from build123d import *

# Parameters (mm, degrees)
SKETCH3_W                = 25.4
SKETCH3_H                = 25.4
SKETCH3_W_2              = 22.225
SKETCH3_H_2              = 22.225
BOSS_EXTRUDE1_DEPTH      = 76.2
BOSS_EXTRUDE1_DEPTH_BACK = 76.2
SKETCH4_W                = 25.4
SKETCH4_H                = 25.4
SKETCH4_W_2              = 22.225
SKETCH4_H_2              = 22.225
CUT_EXTRUDE1_DEPTH       = 7.9375


with BuildPart() as part:
    # Sketch3 → Boss-Extrude1 (new body, two sides)
    with BuildSketch(Plane.XY) as boss_extrude1_sk:
        Rectangle(SKETCH3_W, SKETCH3_H)
        Rectangle(SKETCH3_W_2, SKETCH3_H_2, mode=Mode.SUBTRACT)
    extrude(amount=BOSS_EXTRUDE1_DEPTH)
    extrude(boss_extrude1_sk.sketch, amount=-BOSS_EXTRUDE1_DEPTH_BACK)

    # Sketch4 → Cut-Extrude1 (cut)
    with BuildSketch(Plane(origin=(0, 0, -76.2), x_dir=(-1, 0, 0), z_dir=(0, 0, -1))):
        Rectangle(SKETCH4_W, SKETCH4_H)
        Rectangle(SKETCH4_W_2, SKETCH4_H_2, mode=Mode.SUBTRACT)
    extrude(amount=-CUT_EXTRUDE1_DEPTH, mode=Mode.SUBTRACT)


solid = part.part
Input: part model. Units: mm. Frame: model coordinates. A direction names the side the tool comes from. Round coordinates to 2 decimals unless told otherwise and drop trailing zeros. Order: outer loops, then holes, each group sorted by start corner. A loop starts at its lowest first (then second) coordinate and runs counter-clockwise, first axis right, second up. Notation, with made-up numbers: (-38, 39.5) - (-20, 39.5) arc R25 cw to (-20, 69.5) - close; hole circle Ø10 at (39, 64). An arc over 180 degrees is marked (long way). Answer as a JSON object with one key per item and string values. Group by question number.
(1) Draft query along Y for faces 1 (the face through (12.7, 0, 5)), 2 (the face through (11.112, 0, 5)), 3 (the face through (0, -12.7, 5)). Return one class per face: released by +Y, released by -Y, zero draft, split by the parting line, or undercut.
(2) Material intervals for probe 1 along X at (y, z) = (0.5, 14), sorted ascending. Write a range as from..to.
(3) Reachability of faces 4 (the face through (0, -11.112, 5)), 5 (the face through (11.3, 0.1, -68.262)) from +Z, -Z, +X, -X, +Y, -Y: full face, straight path, thin tool, end or side. Return the list, or none.
(4) Cut plane C-C (z = 24.5). Return loops of the section in (x, y).
(5) Cut plane A-A (x = -1.25). Return loops of the section in (y, z), then the cut area to 3 significant figures.
Here are the results:
{
 "1": {"face 1": "zero draft", "face 2": "undercut", "face 3": "released by -Y"},
 "2": {"probe 1": "x = -12.7..-11.11, 11.11..12.7"},
 "3": {"face 4": "+Z, -Z", "face 5": "-Z, +X, -X, +Y, -Y"},
 "4": {"outline": "(-12.7, -12.7) - (12.7, -12.7) - (12.7, 12.7) - (-12.7, 12.7) - close; hole (-11.11, -11.11) - (11.11, -11.11) - (11.11, 11.11) - (-11.11, 11.11) - close"},
 "5": {"outline": "(-12.7, -68.26) - (-11.11, -68.26) - (-11.11, 76.2) - (-12.7, 76.2) - close; (11.11, -68.26) - (12.7, -68.26) - (12.7, 76.2) - (11.11, 76.2) - close", "area": "459 mm^2"}
}
